from build123d import *

# Parameters (mm, degrees)
SKETCH1_W                                            = 45
SKETCH1_H                                            = 33
BOSS_EXTRUDE1_DEPTH                                  = 45
CUT_EXTRUDE1_DEPTH                                   = 45
CSK_FOR_M5_COUNTERSUNK_RAISED_HEAD_SCREW_D           = 5.5
CSK_FOR_M5_COUNTERSUNK_RAISED_HEAD_SCREW_DEPTH       = 12
CSK_FOR_M5_COUNTERSUNK_RAISED_HEAD_SCREW_CSINK_D     = 10.4
CSK_FOR_M5_COUNTERSUNK_RAISED_HEAD_SCREW_CSINK_ANGLE = 90
CSK_FOR_M5_COUNTERSUNK_RAISED_HEAD_SCREW_TIP         = 1.652366702


with BuildPart() as part:
    # Sketch1 → Boss-Extrude1 (new body)
    with BuildSketch(Plane.XY):
        Rectangle(SKETCH1_W, SKETCH1_H)
    extrude(amount=BOSS_EXTRUDE1_DEPTH)

    # Sketch2 → Cut-Extrude1 (cut)
    with BuildSketch(Plane.XY.offset(45)):
        with BuildLine():
            Line((-5, -9.744997998), (-10.668119688, -16.5))
            Line((-10.668119688, -16.5), (10.668119688, -16.5))
            Line((10.668119688, -16.5), (5, -9.744997998))
            ThreePointArc((5, -9.744997998), (0, 4.5), (-5, -9.744997998))
        make_face()
    extrude(amount=-CUT_EXTRUDE1_DEPTH, mode=Mode.SUBTRACT)

    # CSK for M5 Countersunk Raised Head Screw1
    with Locations(Plane(origin=(0, 16.5, 0), x_dir=(1, 0, 0), z_dir=(0, 1, 0))):
        with Locations((-16, -37.5), (-16, -7.5), (16, -7.5), (16, -37.5)):
            CounterSinkHole(CSK_FOR_M5_COUNTERSUNK_RAISED_HEAD_SCREW_D / 2, CSK_FOR_M5_COUNTERSUNK_RAISED_HEAD_SCREW_CSINK_D / 2, depth=CSK_FOR_M5_COUNTERSUNK_RAISED_HEAD_SCREW_DEPTH, counter_sink_angle=CSK_FOR_M5_COUNTERSUNK_RAISED_HEAD_SCREW_CSINK_ANGLE)
            with Locations((0, 0, -(CSK_FOR_M5_COUNTERSUNK_RAISED_HEAD_SCREW_DEPTH + CSK_FOR_M5_COUNTERSUNK_RAISED_HEAD_SCREW_TIP / 2))):  # 118° drill point
                Cone(0, CSK_FOR_M5_COUNTERSUNK_RAISED_HEAD_SCREW_D / 2, CSK_FOR_M5_COUNTERSUNK_RAISED_HEAD_SCREW_TIP, mode=Mode.SUBTRACT)


solid = part.part
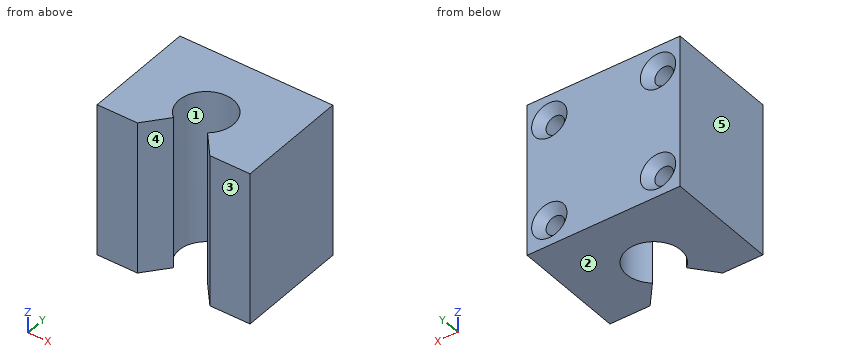
Part model, mm, in its own coordinate system. Face numbers are marked on the shaded views. A direction names the side the tool comes from. Give positions to 0.01 mm unless a question says otherwise; leave off trailing zeros. Order: outer loops, then holes, each group sorted by start corner. A loop starts at its lowest first (then second) coordinate and runs counter-clockwise, first axis right, second up. Notation, with made-up numbers: (-28.75, 22.5) - (27.25, 22.5) arc R22 ccw to (27.25, 42.5) - close; hole circle Ø11 at (-38, -16.5). An arc over 180 degrees is marked (long way). Use a Markdown table: item, result.
1) Flat gauge pins, fed straight in: P1, Ø9.5, axis at x = 0, y = -3.5, coming from the +Z side; P2, Ø4.5, axis at x = 16, z = 7.5, coming from the +Y side. Where does each tip first touch, or does it go through?
Checked values:
| item | result |
|---|---|
| P1 | through |
| P2 | y = 4.2 |
2) Two-plate mould, pull along Y, no slides. Class the marked faces 1, 2 and 3: +Y half, -Y half, draft (parallel to the pull), parting line (faces both ways), or undercut.
Checked values:
| item | result |
|---|---|
| face 1 | undercut |
| face 2 | draft |
| face 3 | -Y half |
3) Saw through at A-A on y = -3.5. List the corners of the cut face in (x, z).
Checked values:
| item | result |
|---|---|
| outline | (-22.5, 0) - (-8, 0) - (-8, 45) - (-22.5, 45) - close; (8, 0) - (22.5, 0) - (22.5, 45) - (8, 45) - close |
4) Saw through at C-C on y = 10. List the corners of the cut face in (x, z).
Checked values:
| item | result |
|---|---|
| outline | (-22.5, 0) - (22.5, 0) - (22.5, 45) - (-22.5, 45) - close; hole circle Ø5.5 at (-16, 7.5); hole circle Ø5.5 at (-16, 37.5); hole circle Ø5.5 at (16, 7.5); hole circle Ø5.5 at (16, 37.5) |
5) Saw through at D-D on z = 24.5. List the corners of the cut face in (x, y) (3 decimals), plus the area to 3 significant figures.
Checked values:
| item | result |
|---|---|
| outline | (-22.5, -16.5) - (-10.668, -16.5) - (-5, -9.745) arc R8 cw (long way) to (5, -9.745) - (10.668, -16.5) - (22.5, -16.5) - (22.5, 16.5) - (-22.5, 16.5) - close |
| area | 1,190 mm² |
6) 3-axis set-ups, long thin cutter, end or side, ignore diameter. For the marked faces 4 and 5: which of +Z, -Z, +X, -X, +Y, -Y reach the whole face in a straight line?
Checked values:
| item | result |
|---|---|
| face 4 | +Z, -Z, -Y |
| face 5 | +Z, -Z, -X, +Y, -Y |
7) Probe L1, parallel to X at y = 7.75, z = 37.5; L2, parallel to Z at x = 16, y = 9; L3, parallel to Z at x = 15, y = 11. List the from-to ranges inside material, lowest first. Write a range as from..to.
Checked values:
| item | result |
|---|---|
| L1 | -22.5..-18.75, -13.25..13.25, 18.75..22.5 |
| L2 | 0..4.75, 10.25..34.75, 40.25..45 |
| L3 | 0..4.94, 10.06..34.94, 40.06..45 |
8) Saw through at B-B on x = -6.5. List the corners of the cut face in (y, z).
Checked values:
| item | result |
|---|---|
| outline | (-11.53, 0) - (-8.16, 0) - (-8.16, 45) - (-11.53, 45) - close; (1.16, 0) - (16.5, 0) - (16.5, 45) - (1.16, 45) - close |
